For this review, take the finished solid that the model builds, in its own axes (mm). A direction names the side the tool comes from. Round coordinates to 2 decimals unless told otherwise and drop trailing zeros. Loops run counter-clockwise (first coordinate to the right, second up) from the corner with the lowest first, then second, coordinate; pieces in that order, holes last.
1. Tool access review of faces 4 (the flat face through (20, 6, 16.5)), 5 (the cylindrical face through (-10.017, 7.07, 1.651)), 6 (the cylindrical face through (-0.434, 6.084, 3.452)), 7 (the flat face through (-15, 6, 5)): name each direction out of +Z, -Z, +X, -X, +Y, -Y from which nothing blocks a thin tool from reaching the whole face with its end or side.
2. Consider section B-B on z = 1.5. State the section outline as (x, y) points, then the cut area to 3 significant figures.
3. Consider section C-C on y = 7. State how many separate pieces and enclosed holes the cut face has, then the cut area to 3 significant figures.
4. Draft analysis for pull direction Z (two halves, no side actions). For faces 1 (the flat face through (10.944, 5.916, -11.324)), 2 (the cylindrical face through (2.106, 7.07, -10.456)), 3 (the flat face through (0, 12, 6)), state which applies: released by +Z, released by -Z, zero draft, split by the parting line, or undercut.
5. Consider section D-D on x = 11. State the section outline as (y, z) points, then the cut area to 3 significant figures.
6. Consider section A-A on x = 23. State the section outline as (y, z) points.
7. To check wall thickness, follow line 1 along X through (y, z) = (9.5, 1.5); line 2 along Z through (x, y) = (0, 6.25); line 3 along Y through (x, z) = (-23, 19). State the ranges of each line that lie inside material, in increasing order.
8. Clearance check with flat-ended pins moving along their axes: pin 1 Ø1.5 at (y, z) = (4.5, -7) entering from +X; pin 2 Ø6 at (x, y) = (23, 6.5) entering from -Z. State where each tip first meets the part, or that it passes through.
from build123d import *

# Parameters (mm, degrees)
BOSS_EXTRUDE1_DEPTH = 12
SKETCH2_R           = 2
CUT_EXTRUDE1_DEPTH  = 39
CUT_EXTRUDE2_DEPTH  = 10
SKETCH3_7_R         = 2
CUT_EXTRUDE3_DEPTH  = 13
CHAMFER1_SIZE       = 1


with BuildPart() as part:
    # Sketch1 → Boss-Extrude1 (new body)
    with BuildSketch(Plane(origin=(0, 0, 0), x_dir=(1, 0, 0), z_dir=(0, 1, 0))):
        Polygon((15, -16.5), (27.5, -16.5), (27.5, -21.5), (-27.5, -21.5), (-27.5, -16.5), (-15, -16.5), (-15, 6.5), (-7, 16.5), (7, 16.5), (15, 6), align=None)
    extrude(amount=BOSS_EXTRUDE1_DEPTH)

    # Sketch2 → Cut-Extrude1 (cut, through all)
    with BuildSketch(Plane.XY.offset(21.5)):
        with Locations((-23, 6)):
            Circle(SKETCH2_R)
        with Locations((23, 6)):
            Circle(SKETCH2_R)
    extrude(amount=-CUT_EXTRUDE1_DEPTH, mode=Mode.SUBTRACT)

    # Sketch3 → Cut-Extrude2 (cut)
    with BuildSketch(Plane(origin=(0, 12, 0), x_dir=(1, 0, 0), z_dir=(0, 1, 0))):
        with BuildLine():
            ThreePointArc((-4.67280566, 11.716690277), (-14.018384458, -1.469804084), (-4.729700131, -14.696437068))
            ThreePointArc((-4.729700131, -14.696437068), (-2.172187792, -13.488492269), (-3.380132591, -10.93097993))
            ThreePointArc((-3.380132591, -10.93097993), (-10.018393738, -1.478420154), (-3.339472326, 7.945454111))
            ThreePointArc((-3.339472326, 7.945454111), (-2.12052091, 10.49773886), (-4.67280566, 11.716690277))
        make_face()
        with BuildLine():
            ThreePointArc((4.729700131, -14.696437068), (2.172187792, -13.488492269), (3.380132591, -10.93097993))
            ThreePointArc((3.380132591, -10.93097993), (10.018393738, -1.478420154), (3.339472326, 7.945454111))
            ThreePointArc((3.339472326, 7.945454111), (2.12052091, 10.49773886), (4.67280566, 11.716690277))
            ThreePointArc((4.67280566, 11.716690277), (14.018384458, -1.469804084), (4.729700131, -14.696437068))
        make_face()
    extrude(amount=-CUT_EXTRUDE2_DEPTH, mode=Mode.SUBTRACT)

    # Sketch3_7 → Cut-Extrude3 (cut, through all)
    with BuildSketch(Plane(origin=(0, 12, 0), x_dir=(1, 0, 0), z_dir=(0, 1, 0))):
        with Locations((0, -1.5)):
            Circle(SKETCH3_7_R)
    extrude(amount=-CUT_EXTRUDE3_DEPTH, mode=Mode.SUBTRACT)

    # Chamfer1
    chamfer1_edges = [part.edges().sort_by_distance(p)[0] for p in [
        (-15, 6, 16.5),
        (15, 6, 16.5),
    ]]
    chamfer(chamfer1_edges, length=CHAMFER1_SIZE)


solid = part.part
Resolved:
1. face 4: -Z, +X, +Y, -Y
1. face 5: +Y
1. face 6: +Y, -Y
1. face 7: -Z, -X, +Y, -Y
2. outline: (-15, 0) - (-2, 0) - (-2, 12) - (-10.02, 12) - (-10.02, 2) - (-14.02, 2) - (-14.02, 12) - (-15, 12) - close; (2, 0) - (15, 0) - (15, 12) - (14.02, 12) - (14.02, 2) - (10.02, 2) - (10.02, 12) - (2, 12) - close
2. area: 232 mm2
3. separate pieces: 3
3. enclosed holes: 3
3. area: 875 mm2
4. face 1: released by -Z
4. face 2: undercut
4. face 3: zero draft
5. outline: (0, -11.25) - (12, -11.25) - (12, -7.19) - (2, -7.19) - (2, 10.19) - (12, 10.19) - (12, 21.5) - (0, 21.5) - close
5. area: 219 mm2
6. outline: (0, 16.5) - (4, 16.5) - (4, 21.5) - (0, 21.5) - close; (8, 16.5) - (12, 16.5) - (12, 21.5) - (8, 21.5) - close
7. line 1: x = -15 to -14.02, -10.02 to -2, 2 to 10.02, 14.02 to 15
7. line 2: z = -16.5 to -0.5, 3.5 to 21.5
7. line 3: y = 0 to 4, 8 to 12
8. pin 1: stops at x = 14.81
8. pin 2: stops at z = 16.5
